Part model, mm, in its own coordinate system. A direction names the side the tool comes from. Round coordinates to 2 decimals unless told otherwise and drop trailing zeros. Write each loop counter-clockwise with the first axis right and the second up, starting at its lowest first coordinate (ties: lowest second). Pieces come first, ordered by that corner, then holes.
Autodesk Inventor part; units mm, degrees
ref_plane "FDT_KSAUFSATZ_XY" through (0, 0, 17) normal (0, 0, 1) x (-1, 0, 0)
ref_plane "FDT_KSAUFSATZ_YZ" through (0, 0, 17) normal (-1, 0, 0) x (0, -1, 0)
ref_plane "FDT_KSAUFSATZ_ZX" through (0, 0, 17) normal (0, -1, 0) x (0, 0, 1)
sketch "Sketch_2" plane through (0, 0, 0) normal (1, 0, 0) x (0, 1, 0)
  line L0 (0, -125) -> (0, 8)
  line L1 (0, 8) -> (6, 8)
  line L2 (6, 8) -> (6, -117)
  line L3 (6, -117) -> (16, -117)
  line L4 (16, -117) -> (16, -125)
  line L5 (16, -125) -> (0, -125)
  line L6 (0, -125) -> (0, 8)
revolve "Revolution1" add sketch "Sketch_2" angle 360 about axis through (0, 0, -125) along (0, 0, -1)
sketch "Sketch_6" plane through (0, 0, 0) normal (1, 0, 0) x (0, 1, 0)
  line L0 (0, 7) -> (0, 30)
  line L1 (0, 30) -> (4.233, 30)
  line L2 (4.233, 30) -> (5, 29.233)
  line L3 (5, 29.233) -> (5, 11.698)
  line L4 (5, 11.698) -> (4.2362, 9.5994)
  arc A0 (4.2362, 9.5994) -> (4.2, 9.3942) centre (4.8, 9.3942) ccw
  line L5 (4.2, 9.3942) -> (4.2, 8.6)
  arc A1 (4.2, 8.6) -> (4.8, 8) centre (4.8, 8.6) ccw
  line L6 (4.8, 8) -> (5, 8)
  line L7 (5, 8) -> (5, 7)
  line L8 (5, 7) -> (0, 7)
  line L9 (0, 7) -> (0, 30)
revolve "Revolution2" add sketch "Sketch_6" angle 360 about axis through (0, 0, 7) along (0, 0, -1)
thread "Thread1"
sketch "Sketch_7" plane through (0, 0, 2) normal (0, 0, 1) x (1, 0, 0)
  line L0 (-10, 20) -> (-10, -10)
  line L1 (-10, -10) -> (-5, -10)
  line L2 (-5, -10) -> (-5, 10)
  line L3 (-5, 10) -> (5, 10)
  line L4 (5, 10) -> (5, -10)
  line L5 (5, -10) -> (10, -10)
  line L6 (10, -10) -> (10, 20)
  line L7 (10, 20) -> (-10, 20)
extrude "Extrusion1" cut sketch "Sketch_7" along normal blind 7
ref_plane "FDT_KSAUFSATZ_XY" through (0, 0, 17) normal (0, 0, 1) x (-1, 0, 0)
ref_plane "FDT_KSAUFSATZ_YZ" through (0, 0, 17) normal (-1, 0, 0) x (0, -1, 0)
ref_plane "FDT_KSAUFSATZ_ZX" through (0, 0, 17) normal (0, -1, 0) x (0, 0, 1)
ref_plane "FDT_NUT_XY" through (0, 0, 17) normal (0, 0, 1) x (-1, 0, 0)
ref_plane "FDT_NUT_YZ" through (0, 0, 17) normal (-1, 0, 0) x (0, -1, 0)
ref_plane "FDT_NUT_ZX" through (0, 0, 17) normal (0, -1, 0) x (0, 0, 1)
ref_plane "KS_XY" through (0, 0, 0) normal (0, 0, -1) x (1, 0, 0)
ref_plane "KS_YZ" through (0, 0, 0) normal (1, 0, 0) x (0, -1, 0)
ref_plane "KS_ZX" through (0, 0, 0) normal (0, -1, 0) x (0, 0, -1)
ref_plane "NUT1_XY" through (0, 0, 22) normal (0, 0, 1) x (1, 0, 0)
ref_plane "NUT1_YZ" through (0, 0, 22) normal (1, 0, 0) x (0, 1, 0)
ref_plane "NUT1_ZX" through (0, 0, 22) normal (0, 1, 0) x (0, 0, 1)
properties part number "193992 DSNU-32-60-PPS---(A---00--0-KS)"
Q1. Which spindle directions (+Z, -Z, +X, -X, +Y, -Y) get a long thin tool onto all of the face, cutting with end or side? Do faces 1 (the flat face through (0, 7, -117)), 2 (the flat face through (5, 0, 5)), 3 (the flat face through (-5, 0, 5)). Say none if no direction does.
Values follow:
face 1: +Z
face 2: +Z, +X, +Y, -Y
face 3: +Z, -X, +Y, -Y
Q2. Mould opens along Z. For faces 4 (the flat face through (0, 0, -125)), 5 (the cylindrical face through (0, -6, -55)), 6 (the cylindrical face through (1.262, 4.006, 8.992)), 7 (the flat face through (3, -4, 8)) say: +Z half, -Z half, draft (parallel to the pull), parting line (faces both ways), or undercut.
Values follow:
face 4: -Z half
face 5: draft
face 6: undercut
face 7: undercut
Q3. Cut at D-D on x = -14. Write the cut outline in (y, z), plus the area to 3 significant figures.
Values follow:
outline: (-7.75, -125) - (7.75, -125) - (7.75, -117) - (-7.75, -117) - close
area: 124 mm2
Q4. Cut at B-B on y = 0. Write the cut outline in (x, z), plus the area to 3 significant figures.
Values follow:
outline: (-16, -125) - (16, -125) - (16, -117) - (6, -117) - (6, 2) - (5, 2) - (5, 8) - (4.8, 8) arc R0.6 cw to (4.2, 8.6) - (4.2, 9.39) arc R0.6 cw to (4.24, 9.6) - (5, 11.7) - (5, 29.23) - (4.23, 30) - (-4.23, 30) - (-5, 29.23) - (-5, 11.7) - (-4.24, 9.6) arc R0.6 cw to (-4.2, 9.39) - (-4.2, 8.6) arc R0.6 cw to (-4.8, 8) - (-5, 8) - (-5, 2) - (-6, 2) - (-6, -117) - (-16, -117) - close
area: 1,960 mm2
Q5. Cut at C-C on z = -87. Write the cut outline in (x, y), plus the area to 3 significant figures.
Values follow:
outline: circle Ø12 at (0, 0)
area: 113 mm2
Q6. Cut at A-A on x = 0. Write the cut outline in (y, z), plus the area to 3 significant figures.
Values follow:
outline: (-16, -125) - (16, -125) - (16, -117) - (6, -117) - (6, 8) - (4.8, 8) arc R0.6 cw to (4.2, 8.6) - (4.2, 9.39) arc R0.6 cw to (4.24, 9.6) - (5, 11.7) - (5, 29.23) - (4.23, 30) - (-4.23, 30) - (-5, 29.23) - (-5, 11.7) - (-4.24, 9.6) arc R0.6 cw to (-4.2, 9.39) - (-4.2, 8.6) arc R0.6 cw to (-4.8, 8) - (-6, 8) - (-6, -117) - (-16, -117) - close
area: 1,970 mm2
Q7. Drop flat-ended pins along their axis: pin 1 (0.5 mm diameter, centred on x = -5.5, y = 1, fed in from +Z); pin 2 (4 mm diameter, centred on x = -5.5, y = 7, fed in from +Z); pin 3 (8 mm diameter, centred on y = -8, z = -108, fed in from +X). Give the stop position or say it passes through.
Values follow:
pin 1: stops at z = 2
pin 2: stops at z = -117
pin 3: stops at x = 4.47
Q8. Wall check: L1, parallel to Z at x = -8, y = 4; L2, parallel to Z at x = 1, y = 5.5; L3, parallel to Y at x = 1.5, z = 18. Give the ranges that are in metal, low to high.
Values follow:
L1: z = -125 to -117
L2: z = -125 to 8
L3: y = -4.77 to 4.77
